Could you check a few things on this model? Use its own coordinates, in mm. A direction names the side the tool comes from. Give positions to 0.01 mm unless a question says otherwise; leave off trailing zeros. Order: outer loops, then holes, each group sorted by start corner. A loop starts at its lowest first (then second) coordinate and runs counter-clockwise, first axis right, second up. Notation, with made-up numbers: (-25.5, -3.5) - (-21.5, -3.5) arc R20 ccw to (-21.5, 4.5) - close; hole circle Ø5 at (76.5, 58.25). An arc over 180 degrees is marked (long way). Put each result on its own line as item: value.
from build123d import *

# Parameters (mm, degrees)
F0_W     = 350
F0_H     = 310
F1_DEPTH = 295
F3_DEPTH = 18
F5_DEPTH = 18


with BuildPart() as f1:
    # F0 (on Front) → F1 (new body)
    with BuildSketch(Plane.XZ):
        with Locations((175, 155)):
            Rectangle(F0_W, F0_H)
    extrude(amount=F1_DEPTH)

    # F2 (on face) → F3 (join)
    with BuildSketch(Plane.XZ.offset(295)):
        with BuildLine():
            ThreePointArc((18.2292630883, 0), (70.1907873154, -30), (122.1523115424, 0))
            Line((122.1523115424, 0), (18.2292630883, 0))
        make_face()
        with BuildLine():
            ThreePointArc((223.2640853139, 0), (275.2256095409, -30), (327.187133768, 0))
            Line((327.187133768, 0), (223.2640853139, 0))
        make_face()
        with BuildLine():
            ThreePointArc((122.1523115424, 0), (128.1463368927, 14.4708572938), (130.1907873154, 30))
            Line((130.1907873154, 30), (10.1907873154, 30))
            ThreePointArc((10.1907873154, 30), (12.235237738, 14.4708572938), (18.2292630883, 0))
            Line((18.2292630883, 0), (122.1523115424, 0))
        make_face()
        with BuildLine():
            ThreePointArc((327.187133768, 0), (333.1811591183, 14.4708572938), (335.2256095409, 30))
            Line((335.2256095409, 30), (215.2256095409, 30))
            ThreePointArc((215.2256095409, 30), (217.2700599636, 14.4708572938), (223.2640853139, 0))
            Line((223.2640853139, 0), (327.187133768, 0))
        make_face()
        with BuildLine():
            Line((10.1907873154, 30), (130.1907873154, 30))
            ThreePointArc((130.1907873154, 30), (70.1907873154, 90), (10.1907873154, 30))
        make_face()
        with BuildLine():
            Line((215.2256095409, 30), (335.2256095409, 30))
            ThreePointArc((335.2256095409, 30), (275.2256095409, 90), (215.2256095409, 30))
        make_face()
    extrude(amount=F3_DEPTH)

    # F4 (on face) → F5 (join)
    with BuildSketch(Plane(origin=(0, 0, 0), x_dir=(-1, 0, 0), z_dir=(0, 1, 0))):
        with BuildLine():
            ThreePointArc((-127.6141306758, 30), (-67.6141306758, -30), (-7.6141306758, 30))
            Line((-7.6141306758, 30), (-127.6141306758, 30))
        make_face()
        with BuildLine():
            Line((-127.6141306758, 30), (-7.6141306758, 30))
            ThreePointArc((-7.6141306758, 30), (-67.6141306758, 90), (-127.6141306758, 30))
        make_face()
        with BuildLine():
            ThreePointArc((-333.5054194927, 30), (-273.5054194927, -30), (-213.5054194927, 30))
            Line((-213.5054194927, 30), (-333.5054194927, 30))
        make_face()
        with BuildLine():
            Line((-333.5054194927, 30), (-213.5054194927, 30))
            ThreePointArc((-213.5054194927, 30), (-273.5054194927, 90), (-333.5054194927, 30))
        make_face()
    extrude(amount=F5_DEPTH)


solid = f1.part
1) Suppose I cut it at B-B, the plane z = 43.5. List the corners of the cut face in (x, y) for me, and give its area (3 significant figures).
Filled in:
outline: (0, -295) - (11.73, -295) - (11.73, -313) - (128.65, -313) - (128.65, -295) - (216.76, -295) - (216.76, -313) - (333.69, -313) - (333.69, -295) - (350, -295) - (350, 0) - (331.97, 0) - (331.97, 18) - (215.04, 18) - (215.04, 0) - (126.08, 0) - (126.08, 18) - (9.15, 18) - (9.15, 0) - (0, 0) - close
area: 112,000 mm^2
2) Suppose I cut it at C-C, the plane y = -147. List the corners of the cut face in (x, z) for me, and give its area (4 significant figures).
Filled in:
outline: (0, 0) - (350, 0) - (350, 310) - (0, 310) - close
area: 108,500 mm^2
3) We'd pull the mould along X, two halves only. Please class faces 1 (the flat face through (0, -145, 153)), 2 (the cylindrical face through (35.358, 8.874, 80.592)), 3 (the flat face through (68, 0, -11)), 4 (the flat face through (350, -145, 153)): pulls with the +X half, pulls with the -X half, needs draft (parallel to the pull), parting line crosses it, or undercut.
Filled in:
face 1: pulls with the -X half
face 2: undercut
face 3: needs draft
face 4: pulls with the +X half
4) I'm going to push flat-ended pins straight in: pin 1 (3 mm diameter, centred on x = 57, y = -266.5, fed in from -Z); pin 2 (5 mm diameter, centred on x = 303.5, z = 271, fed in from +Y). Where does each tip first touch, or does it pass through?
Filled in:
pin 1: stops at z = 0
pin 2: stops at y = 0
5) Suppose I cut it at A-A, the plane x = 110. List the corners of the cut face in (y, z) for me.
Filled in:
outline: (-313, -14.89) - (-295, -14.89) - (-295, 0) - (0, 0) - (0, -12.47) - (18, -12.47) - (18, 72.47) - (0, 72.47) - (0, 310) - (-295, 310) - (-295, 74.89) - (-313, 74.89) - close
6) Which directions (+Z, -Z, +X, -X, +Y, -Y) give clear straight access to the entire face, cutting with the end or side of a thin tool? Please do faces 5 (the flat face through (274, -295, -11)), 6 (the cylindrical face through (333.447, 8.874, 32.638)), 7 (the flat face through (69, -313, 31)).
Filled in:
face 5: -Z, +X, -X
face 6: +Y
face 7: +Z, -Z, +X, -X, -Y
7) Suppose I cut it at D-D, the plane z = 268.5. List the corners of the cut face in (x, y) for me.
Filled in:
outline: (0, -295) - (350, -295) - (350, 0) - (0, 0) - close
8) If I drill on line 1 (Y direction, x = 17, z = 162); line 2 (Z direction, x = 57.5, y = -227), over which ranges is the centre line in solid material (lowest first)? Write a range as [from, to].
Filled in:
line 1: y = [-295, 0]
line 2: z = [0, 310]
